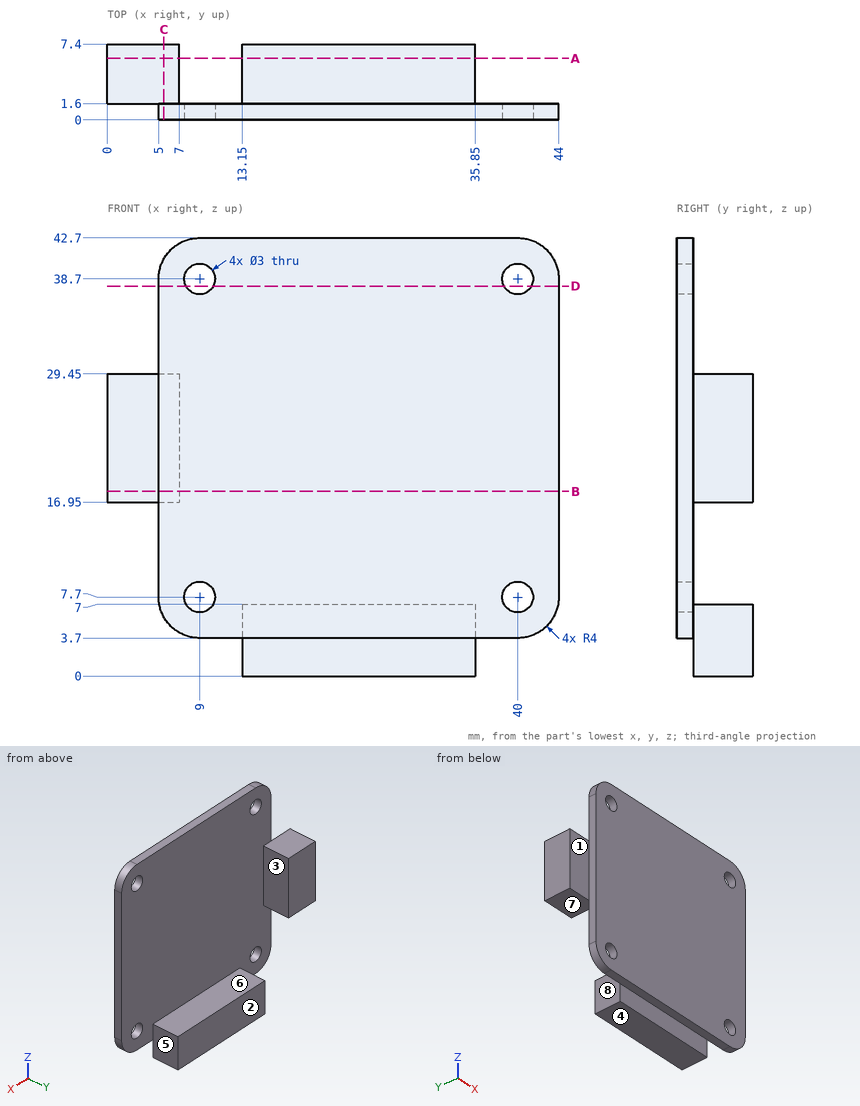
Design review of the part shown in the three views and the two pictorial views. Dimensions are in mm from the part's minimum x, y and z. A direction names the side the tool comes from. Round coordinates to 2 decimals unless told otherwise and drop trailing zeros. Write each loop counter-clockwise with the first axis right and the second up, starting at its lowest first coordinate (ties: lowest second). Pieces come first, ordered by that corner, then holes. Notation, with made-up numbers: (82.5, 52) - (119.5, 52) arc R23 cw to (119.5, 81) - close; hole circle Ø1 at (59, 79). An arc over 180 degrees is marked (long way). Write item = value, one per line. Start each with the question number.
1. For pin 1 Ø1.8 at (x, z) = (25.5, 1.5) entering from -Y; pin 2 Ø3 at (x, y) = (29.5, 5.5) entering from +Z; pin 3 Ø3.5 at (x, z) = (40, 38.7) entering from +Y; pin 4 Ø2.5 at (x, z) = (40, 7.7) entering from -Y, all flat-tipped, find the tip position at first contact; note any pin that passes through.
2. Wall thickness on L1, parallel to X at y = 0.9, z = 7.7; L2, parallel to Z at x = 41, y = 0.5; L3, parallel to X at y = 2.25, z = 20.5: over which ranges is each line inside the solid? List them lowest first.
3. Consider section D-D on z = 38. State the section outline as (x, y) points.
4. Consider section A-A on y = 6. State the section outline as (x, z) points.
5. Consider section B-B on z = 18. State the section outline as (x, y) points.
6. For the marked faces 4, 5, 6, 7 and 8, list the 3-axis set-ups (+Z, -Z, +X, -X, +Y, -Y) from which the entire face can be reached by the end or side of a thin tool; tool diameter is ignored.
7. Draft analysis for pull direction Y (two halves, no side actions). For the marked faces 1, 2 and 3, state which applies: released by +Y, released by -Y, zero draft, split by the parting line, or undercut.
8. Consider section C-C on x = 5.5. State the section outline as (y, z) points, plus the area to 3 significant figures.
Evaluation:
q1.pin_1 = 1.6
q1.pin_2 = 7
q1.pin_3 = 1.6
q1.pin_4 = through
q2.L1 = 5 to 7.5, 10.5 to 38.5, 41.5 to 44
q2.L2 = 3.83 to 6.58, 8.82 to 37.58, 39.82 to 42.57
q2.L3 = 0 to 7
q3.outline = (5, 0) - (7.67, 0) - (7.67, 1.6) - (5, 1.6) - close; (10.33, 0) - (38.67, 0) - (38.67, 1.6) - (10.33, 1.6) - close; (41.33, 0) - (44, 0) - (44, 1.6) - (41.33, 1.6) - close
q4.outline = (0, 16.95) - (7, 16.95) - (7, 29.45) - (0, 29.45) - close; (13.15, 0) - (35.85, 0) - (35.85, 7) - (13.15, 7) - close
q5.outline = (0, 1.6) - (5, 1.6) - (5, 0) - (44, 0) - (44, 1.6) - (7, 1.6) - (7, 7.4) - (0, 7.4) - close
q6.face_4 = -Z, +X, -X, +Y, -Y
q6.face_5 = +Z, -Z, +X, +Y
q6.face_6 = +Z, +X, -X, +Y
q6.face_7 = -Z, +X, -X, +Y
q6.face_8 = +Z, -Z, -X, +Y
q7.face_1 = released by -Y
q7.face_2 = released by +Y
q7.face_3 = zero draft
q8.outline = (0, 5.76) - (1.6, 5.76) - (1.6, 16.95) - (7.4, 16.95) - (7.4, 29.45) - (1.6, 29.45) - (1.6, 40.64) - (0, 40.64) - close
q8.area = 128 mm2
